Input: part model. Units: mm. Frame: model coordinates. Face numbers are marked on the shaded views. Round coordinates to 2 decimals unless told otherwise and drop trailing zeros. Order: outer loops, then holes, each group sorted by start corner. A loop starts at its lowest first (then second) coordinate and runs counter-clockwise, first axis right, second up. Notation, with made-up numbers: (56.5, 21) -> (68.5, 21) arc R25 cw to (68.5, 48) -> close; hole circle Ø5 at (74.25, 51.5). An arc over 180 degrees is marked (long way). Use a Markdown table: item, result.
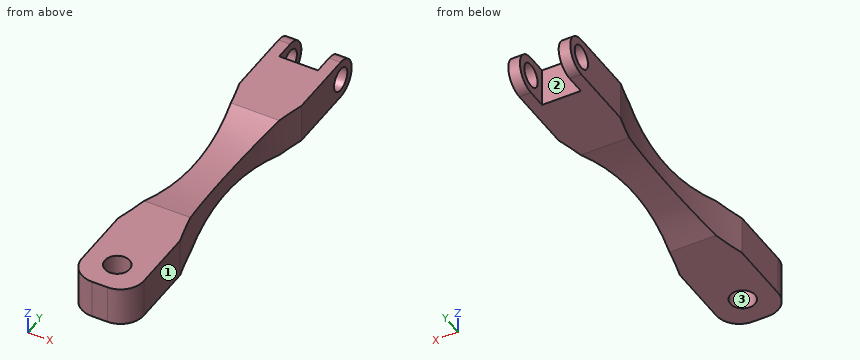
from build123d import *

# Parameters (mm, degrees)
SKETCH1_R           = 1.6
BOSS_EXTRUDE1_DEPTH = 5
SKETCH2_W           = 5
SKETCH2_H           = 5
CUT_EXTRUDE1_DEPTH  = 11
FILLET4_RADIUS      = 2.5
FILLET4_LENGTH      = 1.5
FILLET5_RADIUS      = 2.5
FILLET5_LENGTH      = 1.5
SKETCH3_R           = 1.5
CUT_EXTRUDE2_DEPTH  = 11
CUT_EXTRUDE3_DEPTH  = 11
CUT_EXTRUDE4_DEPTH  = 11


with BuildPart() as part:
    # Sketch1 → Boss-Extrude1 (new body)
    with BuildSketch(Plane.XY):
        with BuildLine():
            Line((-1, -25), (1, -25))
            ThreePointArc((1, -25), (3.121320344, -24.121320344), (4, -22))
            Line((4, -22), (4, 25))
            Line((4, 25), (-4, 25))
            Line((-4, 25), (-4, -22))
            ThreePointArc((-4, -22), (-3.121320344, -24.121320344), (-1, -25))
        make_face()
        with Locations((0, -21)):
            Circle(SKETCH1_R, mode=Mode.SUBTRACT)
    extrude(amount=BOSS_EXTRUDE1_DEPTH)

    # Sketch2 → Cut-Extrude1 (cut)
    with BuildSketch(Plane.XY.offset(5)):
        with Locations((0, 22.5)):
            Rectangle(SKETCH2_W, SKETCH2_H)
    extrude(amount=-CUT_EXTRUDE1_DEPTH, mode=Mode.SUBTRACT)

    # Fillet4: full round fillet: the end face becomes a half cylinder, R = half its width
    fillet4_face = Plane((-3.25, 25, 2.5), x_dir=(-1, 0, 0), z_dir=(0, 1, 0))  # on the end face: x along it, z out of the body
    fillet4_slab = fillet4_face.offset(-FILLET4_RADIUS / 2) * Box(FILLET4_LENGTH, 2 * FILLET4_RADIUS, FILLET4_RADIUS, mode=Mode.PRIVATE)  # the body's end, R deep
    fillet4_round = Plane((-3.25, 22.5, 2.5), x_dir=(0, 1, 0), z_dir=(-1, 0, 0)) * Cylinder(FILLET4_RADIUS, FILLET4_LENGTH, mode=Mode.PRIVATE)  # its axis R under the face
    add(fillet4_slab - fillet4_round, mode=Mode.SUBTRACT)

    # Fillet5: full round fillet: the end face becomes a half cylinder, R = half its width
    fillet5_face = Plane((3.25, 25, 2.5), x_dir=(1, 0, 0), z_dir=(0, 1, 0))  # on the end face: x along it, z out of the body
    fillet5_slab = fillet5_face.offset(-FILLET5_RADIUS / 2) * Box(FILLET5_LENGTH, 2 * FILLET5_RADIUS, FILLET5_RADIUS, mode=Mode.PRIVATE)  # the body's end, R deep
    fillet5_round = Plane((3.25, 22.5, 2.5), x_dir=(0, 1, 0), z_dir=(1, 0, 0)) * Cylinder(FILLET5_RADIUS, FILLET5_LENGTH, mode=Mode.PRIVATE)  # its axis R under the face
    add(fillet5_slab - fillet5_round, mode=Mode.SUBTRACT)

    # Sketch3 → Cut-Extrude2 (cut)
    with BuildSketch(Plane(origin=(4, 0, 0), x_dir=(0, 0, -1), z_dir=(1, 0, 0))):
        with Locations((-2.5, 22.5)):
            Circle(SKETCH3_R)
    extrude(amount=-CUT_EXTRUDE2_DEPTH, mode=Mode.SUBTRACT)

    # Sketch4 → Cut-Extrude3 (cut)
    with BuildSketch(Plane(origin=(4, 0, 0), x_dir=(0, 0, -1), z_dir=(1, 0, 0))):
        with BuildLine():
            Line((-5.938187825, 13.381747244), (-5.854447702, -12.661430853))
            add(Edge.make_bspline(
                [(-5.938187825, 13.381747244), (-1.624651823, 0.354662238), (-5.854447702, -12.661430853)],
                knots=[0, 0, 0, 1, 1, 1], degree=2))
        make_face()
        with BuildLine():
            Line((0.938187825, 13.381747244), (0.854447702, -12.661430853))
            add(Edge.make_bspline(
                [(0.938187825, 13.381747244), (-3.375348177, 0.354662238), (0.854447702, -12.661430853)],
                knots=[0, 0, 0, 1, 1, 1], degree=2))
        make_face()
    extrude(amount=-CUT_EXTRUDE3_DEPTH, mode=Mode.SUBTRACT)

    # Sketch5 → Cut-Extrude4 (cut)
    with BuildSketch(Plane.XY.offset(5)):
        with BuildLine():
            Line((-5.246369121, -17.605604068), (-4.943693979, 16.596686929))
            add(Edge.make_bspline(
                [(-4.943693979, 16.596686929), (1.055826259, -0.52557817), (-5.246369121, -17.605604068)],
                knots=[0, 0, 0, 1, 1, 1], degree=2))
        make_face()
        with BuildLine():
            Line((5.246369121, -17.605604068), (4.943693979, 16.596686929))
            add(Edge.make_bspline(
                [(4.943693979, 16.596686929), (-1.055826259, -0.52557817), (5.246369121, -17.605604068)],
                knots=[0, 0, 0, 1, 1, 1], degree=2))
        make_face()
    extrude(amount=-CUT_EXTRUDE4_DEPTH, mode=Mode.SUBTRACT)


solid = part.part
1) Cut plane A-A on y = -21. Return loops of the section in (x, z), and give its area (3 significant figures).
Answer key:
| item | result |
|---|---|
| outline | (-4, 0) -> (-1.6, 0) -> (-1.6, 5) -> (-4, 5) -> close; (1.6, 0) -> (4, 0) -> (4, 5) -> (1.6, 5) -> close |
| area | 24.0 mm^2 |
2) Draft query along Y for the marked faces 1, 2 and 3. Return one class per face: released by +Y, released by -Y, zero draft, split by the parting line, or undercut.
Answer key:
| item | result |
|---|---|
| face 1 | zero draft |
| face 2 | released by +Y |
| face 3 | undercut |
3) Contact query for flat-ended pins moving along their axis: P1, Ø4, axis at x = 1, y = -6.5, coming from the +Z side; P2, Ø1, axis at x = -1, y = 3.5, coming from the +Z side; P3, Ø2.5, axis at x = -0.5, z = 3, coming from the +Y side; P4, Ø1.8, axis at y = 22.5, z = 2.5, coming from the +X side. Output: stop coordinate, or through.
Answer key:
| item | result |
|---|---|
| P1 | stops at z = 4.72 |
| P2 | stops at z = 3.94 |
| P3 | stops at y = 20 |
| P4 | passes through |
4) Ray query, probe 1 along Y at (x, z) = (-1.25, 1.7); probe 2 along Y at (x, z) = (0, 3.6); probe 3 along X at (y, z) = (-20, 1.6). Return the intervals inside material, ascending.
Answer key:
| item | result |
|---|---|
| probe 1 | y = -24.99 to -22, -20 to 20 |
| probe 2 | y = -25 to -22.6, -19.4 to 20 |
| probe 3 | x = -4 to -1.25, 1.25 to 4 |
5) Cut plane B-B on z = 2.5. State how many separate pieces and enclosed holes the cut face has, and give its area (3 significant figures).
Answer key:
| item | result |
|---|---|
| separate pieces | 3 |
| enclosed holes | 1 |
| area | 282 mm^2 |
